Autodesk Inventor part; units mm, degrees
ref_plane "YZ Plane" through (0, 0, 0) normal (1, 0, 0) x (0, 1, 0)
ref_plane "XZ Plane" through (0, 0, 0) normal (0, 1, 0) x (-1, 0, 0)
ref_plane "XY Plane" through (0, 0, 0) normal (0, 0, 1) x (1, 0, 0)
sketch "Skizze1" plane through (0, 0, 0) normal (1, 0, 0) x (0, 1, 0)
  line L0 (-155, -55) -> (155, -55)
  line L1 (155, -55) -> (155, 55)
  line L2 (155, 55) -> (-155, 55)
  line L3 (-155, 55) -> (-155, -55)
  line L4 (-155, -55) -> (155, 55) construction
  line L5 (155, -55) -> (-155, 55) construction
  point P0 (0, 0)
  dimension "d43" = 310
  dimension "d44" = 110
extrude "Grundlörper" add sketch "Skizze1" along normal blind 5
sketch "Skizze5" plane through (5, 0, 0) normal (1, 0, 0) x (0, 0, -1)
  line L0 (-55, -155) -> (55, -155) construction
  line L1 (-55, 155) -> (-55, -155) construction
  line L2 (55, 155) -> (-55, 155) construction
  line L3 (-91, 0) -> (91, 0) construction
  line L4 (0, -217) -> (0, 217) construction
  line L5 (-55, -30) -> (-30, -30)
  line L6 (-30, -30) -> (-30, 30)
  line L7 (-30, 30) -> (-55, 30)
  line L8 (-55, -30) -> (-55, 30)
  point P0 (0, 0)
  dimension "d50" = 60
  dimension "d51" = 25
extrude "Aussschnitt" cut sketch "Skizze5" against normal through all
sketch "Skizze7" plane through (5, 0, 0) normal (1, 0, 0) x (0, 0, -1)
  line L0 (-77, 0) -> (77, 0)
  line L1 (-55, -145) -> (55, -145) construction
  line L2 (55, -155) -> (55, 155) construction
  line L3 (-55, -155) -> (55, -155) construction
  line L4 (-55, -30) -> (-55, -155) construction
  line L5 (-55, 145) -> (55, 145) construction
  point P0 (0, 0)
  point P1 (-45, -145)
  point P2 (-25, -145)
  point P3 (-5, -145)
  point P4 (15, -145)
  point P5 (35, -145)
  point P6 (-45, -115)
  point P7 (-45, -85)
  point P8 (-45, -55)
  point P9 (-25, -145)
  point P10 (-25, -115)
  point P11 (-25, -85)
  point P12 (-25, -55)
  point P13 (-45, 145)
  point P14 (-25, 145)
  point P15 (-5, 145)
  point P16 (15, 145)
  point P17 (35, 145)
  point P18 (-45, 115)
  point P19 (-45, 85)
  point P20 (-45, 55)
  point P21 (-25, 145)
  point P22 (-25, 115)
  point P23 (-25, 85)
  point P24 (-25, 55)
  dimension "d104" = 10
  dimension "d105" = 10
  dimension "d108" = 20
  dimension "d115" = 30
  dimension "d118" = 20
hole "Bohrung4" at (5, -145, 45) at (5, -145, 25) at (5, -145, 5) at (5, -145, -15) at (5, -145, -35) at (5, -115, 45) at (5, -85, 45) at (5, -55, 45) at (5, -115, 25) at (5, -85, 25) at (5, -55, 25) at (5, 55, 25) at (5, 85, 25) at (5, 115, 25) at (5, 145, 25) at (5, 55, 45) at (5, 85, 45) at (5, 115, 45) at (5, 145, -35) at (5, 145, -15) at (5, 145, 5) at (5, 145, 45) direction (-1, 0, 0) diameter 5.5 end through all
properties part number "200-40-BOGIE-CONNECTOR-06" material "Aluminium 6061"
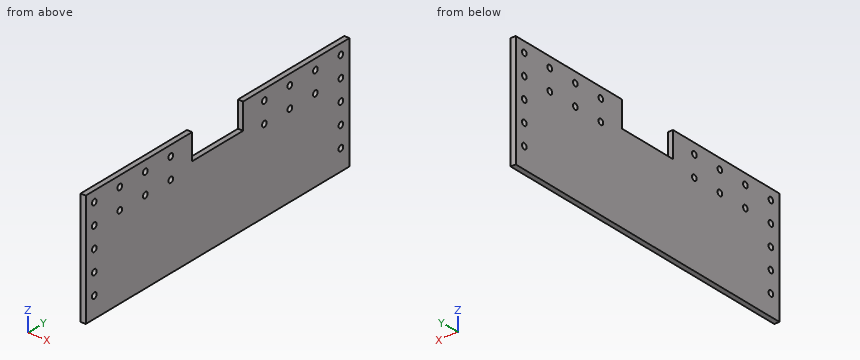
Part model, mm, in its own coordinate system. Coordinates: 2 decimals unless noted, no trailing zeros. Order: outer loops, then holes, each group sorted by start corner. A loop starts at its lowest first (then second) coordinate and runs counter-clockwise, first axis right, second up. Notation, with made-up numbers: M 71,38.5 L 105,38.5 A18 ccw 105,66.5 Z; hole C 55,81.25 d8. An arc over 180 degrees is marked long. Use a Markdown table: item, result.
(1) Cut at C-C on y = 145. Write the cut outline in (x, z), then the cut area to 4 significant figures.
A:
| item | result |
|---|---|
| outline | M 0,-55 L 5,-55 L 5,-37.75 L 0,-37.75 Z; M 0,-32.25 L 5,-32.25 L 5,-17.75 L 0,-17.75 Z; M 0,-12.25 L 5,-12.25 L 5,2.25 L 0,2.25 Z; M 0,7.75 L 5,7.75 L 5,22.25 L 0,22.25 Z; M 0,27.75 L 5,27.75 L 5,42.25 L 0,42.25 Z; M 0,47.75 L 5,47.75 L 5,55 L 0,55 Z |
| area | 412.5 mm^2 |
(2) Cut at A-A on y = 85. Write the cut outline in (x, z), then the cut area to 3 significant figures.
A:
| item | result |
|---|---|
| outline | M 0,-55 L 5,-55 L 5,22.25 L 0,22.25 Z; M 0,27.75 L 5,27.75 L 5,42.25 L 0,42.25 Z; M 0,47.75 L 5,47.75 L 5,55 L 0,55 Z |
| area | 495 mm^2 |
(3) Probe L1, parallel to Z at x = 1.6, y = -115; L2, parallel to Y at x = 2.9, z = -35; L3, parallel to Z at x = 3.9, y = 145. List the from-to ranges inside material, lowest first.
A:
| item | result |
|---|---|
| L1 | z = -55 to 22.25, 27.75 to 42.25, 47.75 to 55 |
| L2 | y = -155 to -147.75, -142.25 to 142.25, 147.75 to 155 |
| L3 | z = -55 to -37.75, -32.25 to -17.75, -12.25 to 2.25, 7.75 to 22.25, 27.75 to 42.25, 47.75 to 55 |
(4) Cut at B-B on z = 5. Write the cut outline in (x, y), then the cut area to 4 significant figures.
A:
| item | result |
|---|---|
| outline | M 0,-155 L 5,-155 L 5,-147.75 L 0,-147.75 Z; M 0,-142.25 L 5,-142.25 L 5,142.25 L 0,142.25 Z; M 0,147.75 L 5,147.75 L 5,155 L 0,155 Z |
| area | 1,495 mm^2 |
(5) Cut at D-D on x = 1.85. State how many separate pieces and enclosed holes the cut face has, then the cut area to 3 significant figures.
A:
| item | result |
|---|---|
| separate pieces | 1 |
| enclosed holes | 22 |
| area | 32,100 mm^2 |
(6) Flat gauge pins, fed straight in: pin 1 (1 mm diameter, centred on y = 24.5, z = -14.5, fed in from -X); pin 2 (4.5 mm diameter, centred on y = 55, z = 25, fed in from -X); pin 3 (2 mm diameter, centred on x = 1.5, y = -3.5, fed in from +Z). Where does each tip first touch, or does it go through?
A:
| item | result |
|---|---|
| pin 1 | stops at x = 0 |
| pin 2 | passes through |
| pin 3 | stops at z = 30 |
